Geometry: final body of the model. Coordinates: model frame, mm. Face numbers are marked on the shaded views. Coordinates: 2 decimals unless noted, no trailing zeros. Loops run counter-clockwise (first coordinate to the right, second up) from the corner with the lowest first, then second, coordinate; pieces in that order, holes last. Notation, with made-up numbers: (17, -16.75) -> (63, -16.75) arc R27 ccw to (63, 13.25) -> close; hole circle Ø2 at (-28, -7.75). An arc over 180 degrees is marked (long way). One line per item, written item: value. Start each with the question number.
Item 1: Section query C-C on z = 31. Return loops of the section in (x, y).
Item 2: Ray query, probe 1 along Y at (x, z) = (-14, 29.5); probe 2 along Z at (x, y) = (-6, 17). Return the intervals inside material, ascending. Write a range as from..to.
Item 3: Mould query, pull axis Y, two halves, no side actions, for the marked faces 1, 2 and 3. Classes: +Y half, -Y half, draft (parallel to the pull), parting line (faces both ways), or undercut.
Item 4: Contact query for a flat-ended pin moving along its axis: pin 1 Ø1.3 at (y, z) = (22.5, 46) entering from -X. Output: stop coordinate, or through.
Item 5: Section query A-A on x = 2. Return loops of the section in (y, z).
Item 6: Section query B-B on y = -17.5. Return loops of the section in (x, z), then the cut area to 3 significant figures.
from build123d import *

# Parameters (mm, degrees)
F0_W      = 50.8
F0_H      = 50.8
F1_DEPTH  = 50.8
F3_T      = -2.54
F2_R      = 11.1895018243
F4_DEPTH  = 2.54
F5_W      = 11.6650760174
F5_H      = 3.2993815839
F6_DEPTH  = 25.4
F7_R      = 2.5171305481
F8_DEPTH  = 25.4
F9_R      = 2.9308146248
F9_R_2    = 3.9125837807
F9_W      = 7.4259676039
F9_H      = 3.2972879708
F10_DEPTH = 25.4


with BuildPart() as f1:
    # F0 (on Top) → F1 (new body)
    with BuildSketch(Plane.XY):
        Rectangle(F0_W, F0_H)
    extrude(amount=F1_DEPTH)

    # F3 (hollow: no face is removed)
    offset(amount=F3_T, mode=Mode.SUBTRACT)

    # F2 (on face) → F4 (cut, through all)
    with BuildSketch(Plane.YZ.offset(25.4)):
        with Locations((0, 32.3844626546)):
            Circle(F2_R)
    extrude(amount=-F4_DEPTH, mode=Mode.SUBTRACT)

    # F5 (on face) → F6 (cut)
    with BuildSketch(Plane(origin=(0, 25.4, 0), x_dir=(-1, 0, 0), z_dir=(0, 1, 0))):
        with Locations((-17.2344464809, 4.7428607941)):
            Rectangle(F5_W, F5_H)
    extrude(amount=-F6_DEPTH, mode=Mode.SUBTRACT)

    # F7 (on face) → F8 (cut)
    with BuildSketch(Plane(origin=(0, 25.4, 0), x_dir=(-1, 0, 0), z_dir=(0, 1, 0))):
        with Locations((-21.0335571319, 45.9851287305)):
            Circle(F7_R)
    extrude(amount=-F8_DEPTH, mode=Mode.SUBTRACT)

    # F9 (on face) → F10 (cut)
    with BuildSketch(Plane(origin=(-25.4, 0, 0), x_dir=(0, -1, 0), z_dir=(-1, 0, 0))):
        with Locations((-21.4459802955, 45.7789190114)):
            Circle(F9_R)
        with Locations((-20.2087108046, 5.3614946082)):
            Circle(F9_R_2)
        with Locations((19.1762130708, 3.9165434428)):
            Rectangle(F9_W, F9_H)
    extrude(amount=-F10_DEPTH, mode=Mode.SUBTRACT)


solid = f1.part
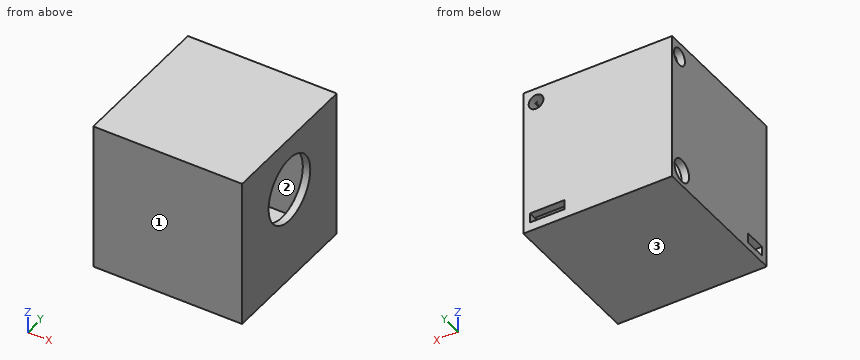
Reply:
1. outline: (-25.4, -25.4) -> (25.4, -25.4) -> (25.4, -11.1) -> (22.86, -11.1) -> (22.86, -22.86) -> (-22.86, -22.86) -> (-22.86, 22.86) -> (22.86, 22.86) -> (22.86, 11.1) -> (25.4, 11.1) -> (25.4, 25.4) -> (-25.4, 25.4) -> close
2. probe 1: y = -25.4..-22.86, 22.86..25.4
2. probe 2: z = 0..2.54, 48.26..50.8
3. face 1: -Y half
3. face 2: undercut
3. face 3: draft
4. pin 1: stops at x = 0
5. outline: (-25.4, 0) -> (25.4, 0) -> (25.4, 50.8) -> (-25.4, 50.8) -> close; hole (-22.86, 2.54) -> (22.86, 2.54) -> (22.86, 48.26) -> (-22.86, 48.26) -> close
6. outline: (-25.4, 0) -> (25.4, 0) -> (25.4, 50.8) -> (-25.4, 50.8) -> (-25.4, 5.57) -> (-22.86, 5.57) -> (-22.86, 48.26) -> (22.86, 48.26) -> (22.86, 2.54) -> (0, 2.54) -> (0, 2.27) -> (-25.4, 2.27) -> close
6. area: 476 mm²
